```python
from build123d import *

# Parameters (mm, degrees)
EXTRUDE_1_DEPTH = 5


with BuildPart() as part:
    # 草图1 → 凸台-拉伸1 (new body)
    with BuildSketch(Plane(origin=(0, 0, 0), x_dir=(1, 0, 0), z_dir=(0, 1, 0))):
        with BuildLine():
            Line((8, 0), (36, 0))
            ThreePointArc((36, 0), (38.828427125, -1.171572875), (40, -4))
            Line((40, -4), (40, -12))
            ThreePointArc((40, -12), (42.343145751, -17.656854249), (48, -20))
            Line((48, -20), (50, -20))
            Line((50, -20), (50, -10))
            Line((50, -10), (55, -10))
            Line((55, -10), (55, 0))
            Line((55, 0), (50, 0))
            Line((50, 0), (50, 10))
            Line((50, 10), (20, 10))
            Line((20, 10), (20, 15))
            Line((20, 15), (10, 15))
            Line((10, 15), (10, 10))
            Line((10, 10), (0, 10))
            Line((0, 10), (0, 8))
            ThreePointArc((0, 8), (2.343145751, 2.343145751), (8, 0))
        make_face()
    extrude(amount=EXTRUDE_1_DEPTH)


solid = part.part
```
Here's how the part is built. I have some questions about the finished solid (model axes, mm). A direction names the side the tool comes from. Give positions to 0.01 mm unless a question says otherwise; leave off trailing zeros. Loops run counter-clockwise (first coordinate to the right, second up) from the corner with the lowest first, then second, coordinate; pieces in that order, holes last. Notation, with made-up numbers: M 85.25,23 L 103.25,23 A31 ccw 103.25,47 Z; hole C 79.25,17 d4. An arc over 180 degrees is marked long. Return JSON: item names as keys, results as strings.
Item 1: Imagine slicing it at C-C on z = 7.5. List the corners of the cut face in (x, y) for me, then the cut area to 3 significant figures.
A:
{"outline": "M 40,0 L 55,0 L 55,5 L 40,5 Z", "area": "75.0 mm^2"}
Item 2: Imagine slicing it at A-A on y = 3.95. List the corners of the cut face in (x, z) for me, then the cut area to 3 significant figures.
A:
{"outline": "M 0,-10 L 10,-10 L 10,-15 L 20,-15 L 20,-10 L 50,-10 L 50,0 L 55,0 L 55,10 L 50,10 L 50,20 L 48,20 A8 ccw 40,12 L 40,4 A4 cw 36,0 L 8,0 A8 ccw 0,-8 Z", "area": "776 mm^2"}
Item 3: Please list where these lines run through material, in increasing order: line 1 (Z direction, x = 16.5, y = 0.4); line 2 (Z direction, x = 33.5, y = 4.35); line 3 (X direction, y = 4.75, z = 10.5).
A:
{"line 1": "z = -15 to 0", "line 2": "z = -10 to 0", "line 3": "x = 40 to 50"}
Item 4: Imagine slicing it at B-B on x = 22. List the corners of the cut face in (y, z) for me.
A:
{"outline": "M 0,-10 L 5,-10 L 5,0 L 0,0 Z"}
Item 5: I'm going to push flat-ended pins straight in: pin 1 Ø2 at (x, y) = (19.5, 3) entering from +Z; pin 2 Ø1.5 at (x, y) = (6, 3) entering from -Z; pin 3 Ø2.5 at (y, z) = (1.5, 7.5) entering from -X. Where does each tip first touch, or does it pass through?
A:
{"pin 1": "stops at z = 0", "pin 2": "stops at z = -10", "pin 3": "stops at x = 40"}
Item 6: On a 3-axis mill with a long thin cutter (end or side, diameter ignored), from which of +Z, -Z, +X, -X, +Y, -Y can I reach the whole of each face in a straight line? I mean faces 1 (the flat face through (40, 2, 8)), 2 (the flat face through (0, 2, -9)), 3 (the flat face through (50, 2, 15)), 4 (the flat face through (10, 2, -13)), 5 (the flat face through (53, 2, 0)). Say none if no direction works.
A:
{"face 1": "+Z, -X, +Y, -Y", "face 2": "+Z, -Z, -X, +Y, -Y", "face 3": "+Z, +X, +Y, -Y", "face 4": "-Z, -X, +Y, -Y", "face 5": "-Z, +X, +Y, -Y"}
